```python
from build123d import *

# Parameters (mm, degrees)
BOSS_EXTRUDE1_DEPTH = 10
CUT_EXTRUDE3_DEPTH  = 8
SKETCH5_R           = 1
CUT_EXTRUDE5_DEPTH  = 7.5
CUT_EXTRUDE7_DEPTH  = 2
CUT_EXTRUDE10_DEPTH = 4
CUT_EXTRUDE12_DEPTH = 7
CUT_EXTRUDE14_DEPTH = 6
CUT_EXTRUDE15_DEPTH = 7
SKETCH18_W          = 1.999299567
SKETCH18_H          = 4.5
CUT_EXTRUDE29_DEPTH = 2
CUT_EXTRUDE30_DEPTH = 2
CUT_EXTRUDE31_DEPTH = 7
CUT_EXTRUDE33_DEPTH = 10


with BuildPart() as part:
    # Sketch1 → Boss-Extrude1 (new body)
    with BuildSketch(Plane.XY):
        Polygon((0, 0), (0, 7), (-3, 7), (-3, 9), (-4.5, 9), (-4.5, 10), (-6, 10), (-6, 0), align=None)
    extrude(amount=BOSS_EXTRUDE1_DEPTH)

    # Sketch3 → Cut-Extrude3 (cut, through all)
    with BuildSketch(Plane(origin=(0, 7, 0), x_dir=(1, 0, 0), z_dir=(0, 1, 0))):
        Polygon((-3, 0), (-3, -1.004111064), (-1, -1.004111064), (-1, -2), (0, -2), (0, 0), align=None)
    extrude(amount=-CUT_EXTRUDE3_DEPTH, mode=Mode.SUBTRACT)

    # Sketch5 → Cut-Extrude5 (cut, symmetric)
    with BuildSketch(Plane(origin=(0, 7, 0), x_dir=(1, 0, 0), z_dir=(0, 1, 0))):
        with Locations((-3, -3.004111064)):
            Circle(SKETCH5_R)
    extrude(amount=CUT_EXTRUDE5_DEPTH, both=True, mode=Mode.SUBTRACT)

    # Sketch7 → Cut-Extrude7 (cut, symmetric)
    with BuildSketch(Plane(origin=(0, 9, 0), x_dir=(1, 0, 0), z_dir=(0, 1, 0))):
        with BuildLine():
            Line((-3, -1.002055532), (-3, -2.004111064))
            ThreePointArc((-3, -2.004111064), (-4, -3.004111064), (-3, -4.004111064))
            Line((-3, -4.004111064), (-3, -10))
            Line((-3, -10), (-5.002055532, -10))
            Line((-5.002055532, -10), (-5.002055532, -3.004111064))
            ThreePointArc((-5.002055532, -3.004111064), (-4.415667043, -1.588444021), (-3, -1.002055532))
        make_face()
    extrude(amount=CUT_EXTRUDE7_DEPTH, both=True, mode=Mode.SUBTRACT)

    # Sketch8 → Cut-Extrude10 (cut)
    with BuildSketch(Plane.ZY.offset(6)):
        Polygon((3, 10), (4, 9), (4, 8), (7, 8), (7, 10), align=None)
    extrude(amount=-CUT_EXTRUDE10_DEPTH, mode=Mode.SUBTRACT)

    # Sketch9 → Cut-Extrude12 (cut, symmetric)
    with BuildSketch(Plane(origin=(-5.002055532, 0, 0), x_dir=(0, 0, -1), z_dir=(1, 0, 0))):
        with BuildLine():
            Line((-8, 9), (-7, 9))
            Line((-7, 9), (-7, 10))
            Line((-7, 10), (-10, 10))
            Line((-10, 10), (-10, 7))
            ThreePointArc((-10, 7), (-9.414213562, 8.414213562), (-8, 9))
        make_face()
        with BuildLine():
            ThreePointArc((-7, 7), (-8, 8), (-9, 7))
            Line((-9, 7), (-7, 7))
        make_face()
        with BuildLine():
            Line((-7, 7), (-9, 7))
            ThreePointArc((-9, 7), (-8, 6), (-7, 7))
        make_face()
    extrude(amount=CUT_EXTRUDE12_DEPTH, both=True, mode=Mode.SUBTRACT)

    # Sketch10 → Cut-Extrude14 (cut)
    with BuildSketch(Plane(origin=(0, 7, 0), x_dir=(1, 0, 0), z_dir=(0, 1, 0))):
        with BuildLine():
            Line((-2, -6), (-3, -6))
            Line((-3, -6), (-3, -8.001400867))
            Line((-3, -8.001400867), (0, -8))
            Line((0, -8), (0, -4))
            ThreePointArc((0, -4), (-1.414213562, -4.585786438), (-2, -6))
        make_face()
    extrude(amount=-CUT_EXTRUDE14_DEPTH, mode=Mode.SUBTRACT)

    # Sketch12 → Cut-Extrude15 (cut, through all)
    with BuildSketch(Plane(origin=(0, 0, 0), x_dir=(0, 0, -1), z_dir=(1, 0, 0))):
        Polygon((-4, 1), (-4, 4), (-8.001400867, 4), (-8, 1), align=None)
    extrude(amount=-CUT_EXTRUDE15_DEPTH, mode=Mode.SUBTRACT)

    # Sketch18 → Cut-Extrude29 (cut)
    with BuildSketch(Plane(origin=(0, 0, 0), x_dir=(0, 0, -1), z_dir=(1, 0, 0))):
        with Locations((-9.000350216, 4.75)):
            Rectangle(SKETCH18_W, SKETCH18_H)
    extrude(amount=-CUT_EXTRUDE29_DEPTH, mode=Mode.SUBTRACT)

    # Sketch21 → Cut-Extrude30 (cut)
    with BuildSketch(Plane.XY.offset(8.000700433)):
        Polygon((0, 6.000000245), (-1.5, 6.000000981), (-1.5, 4), (0, 4), align=None)
    extrude(amount=-CUT_EXTRUDE30_DEPTH, mode=Mode.SUBTRACT)

    # Sketch22 → Cut-Extrude31 (cut)
    with BuildSketch(Plane(origin=(0, 7, 0), x_dir=(1, 0, 0), z_dir=(0, 1, 0))):
        Polygon((0, -4), (-4, -10), (0, -10), align=None)
    extrude(amount=-CUT_EXTRUDE31_DEPTH, mode=Mode.SUBTRACT)

    # Sketch23 → Cut-Extrude33 (cut)
    with BuildSketch(Plane(origin=(0, 7, 0), x_dir=(1, 0, 0), z_dir=(0, 1, 0))):
        with BuildLine():
            Line((-3.002055532, -8), (-0.668346428, -8))
            Line((-0.668346428, -8), (-0.668346428, -10.987104512))
            Line((-0.668346428, -10.987104512), (-5.156575053, -10.987104512))
            Line((-5.156575053, -10.987104512), (-5.002055532, -10))
            ThreePointArc((-5.002055532, -10), (-3.587841969, -9.414213562), (-3.002055532, -8))
        make_face()
    extrude(amount=-CUT_EXTRUDE33_DEPTH, mode=Mode.SUBTRACT)


solid = part.part
```
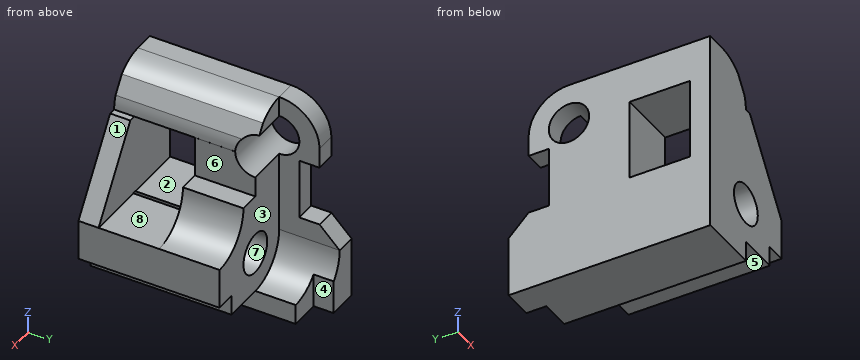
CAD build for the part. Positions are in the model's coordinates, mm. Face numbers are marked on the shaded views. A direction names the side the tool comes from. Round coordinates to 2 decimals unless told otherwise and drop trailing zeros. Write each loop counter-clockwise with the first axis right and the second up, starting at its lowest first coordinate (ties: lowest second). Pieces come first, ordered by that corner, then holes. Notation, with made-up numbers: (50, 30) - (83, 30) arc R13 cw to (83, 50) - close; hole circle Ø5 at (-39.5, -19.5). An arc over 180 degrees is marked (long way). Write item = value, one per line. Start each with the question number.
Q1. Which spindle directions (+Z, -Z, +X, -X, +Y, -Y) get a long thin tool onto all of the face, cutting with end or side? Do the marked faces 1, 2, 3, 4 and 5. Say none if no direction does.
Q2. Probe L1, parallel to Z at x = -5.15, y = 7; L2, parallel to Y at x = -3.75, z = 4.75; L3, parallel to Y at x = -0.5, z = 3.75. List the from-to ranges inside material, lowest first. Write a range as from..to.
Q3. Band-saw the part on A-A (y = 6.75). Give the cut face in (x, z).
Q4. Band-saw the part on D-D (y = 2). Give the cut face in (x, z).
Q5. Mould opens along X. For the marked faces 6, 7 and 8 say: pulls with the +X half, pulls with the -X half, needs draft (parallel to the pull), parting line crosses it, or undercut.
Q6. Drop flat-ended pins along their axis: pin 1 (0.8 mm diameter, centred on y = 6, z = 0.5, fed in from +X); pin 2 (0.8 mm diameter, centred on x = -5.5, z = 5, fed in from +Y); pin 3 (3 mm diameter, centred on x = -5, z = 8.5, fed in from +Y); pin 4 (1.2 mm diameter, centred on x = -3, z = 3, fed in from +Y). Give the stop position or say it passes through.
Q7. Band-saw the part on B-B (z = 8.5). Give the cut face in (x, y).
Answers below:
q1.face_1 = +Z, +X, +Y, -Y
q1.face_2 = +X, -X
q1.face_3 = +Z, +X, +Y
q1.face_4 = +Z, -Z, +X, +Y
q1.face_5 = -Z, +X, +Y, -Y
q2.L1 = 0..7, 9..10
q2.L2 = 0..1, 4..7
q2.L3 = 0..7
q3.outline = (-6, 0) - (-3, 0) - (-3, 1) - (-1, 1) - (-1, 2) - (0, 2) - (0, 4) arc R2 cw to (-2, 6) - (-3, 6) - (-3, 7.03) - (-6, 7.03) - close; (-6, 8.97) - (-3.31, 8.97) - (-3.65, 9.47) arc R2 ccw to (-5, 10) - (-6, 10) - close; hole circle Ø2 at (-3, 3)
q4.outline = (-6, 0) - (-3, 0) - (-3, 1) - (-1, 1) - (-1, 2) - (0, 2) - (0, 4) - (-2.91, 4) arc R1 cw (long way) to (-3.09, 4) - (-6, 4) - close; (-6, 8) - (-3, 8) arc R2 ccw to (-3.12, 8.68) - (-3.65, 9.47) arc R2 ccw to (-5, 10) - (-6, 10) - close
q5.face_6 = pulls with the +X half
q5.face_7 = undercut
q5.face_8 = needs draft
q6.pin_1 = -3
q6.pin_2 = 8
q6.pin_3 = 9
q6.pin_4 = through
q7.outline = (-6, 0) - (-3.07, 0) - (-3.07, 6.13) - (-6, 6.13) - close; (-6, 7.87) - (-5, 7.87) - (-5, 8.94) - (-6, 8.94) - close
